Work out the finished part from the listing and answer in its coordinate system (mm). A direction names the side the tool comes from. Round coordinates to 2 decimals unless told otherwise and drop trailing zeros. Order: outer loops, then holes, each group sorted by start corner. A loop starts at its lowest first (then second) coordinate and runs counter-clockwise, first axis right, second up. Notation, with made-up numbers: (-27, 84.25) - (1, 84.25) arc R20 ccw to (1, 103.25) - close; hole circle Ø7 at (10, 38). An arc over 180 degrees is marked (long way). Put each result on its own line as item: value.
```python
from build123d import *

# Parameters (mm, degrees)
BOSS_EXTRU_1_DEPTH           = 22.5
R_P_TITION_CIRCULAIRE2_COUNT = 3
TROU_TARAUD_M51_D            = 4.2
TROU_TARAUD_M51_DEPTH        = 14
TROU_TARAUD_M51_TIP          = 1.2618073
TROU_TARAUD_M52_D            = 4.2
TROU_TARAUD_M52_DEPTH        = 14
TROU_TARAUD_M52_TIP          = 1.2618073
ESQUISSE6_R                  = 4
ESQUISSE6_R_2                = 2.807618462
BOSS_EXTRU_2_DEPTH           = 15


with BuildPart() as part:
    # Esquisse1 → Boss.-Extru.1 (new body, symmetric)
    with BuildSketch(Plane.XY):
        with BuildLine():
            Line((0, 0), (-3.464101615, 2))
            ThreePointArc((-3.464101615, 2), (-2.618614683, 3.023715784), (-1.484614978, 3.714285714))
            ThreePointArc((-1.484614978, 3.714285714), (-1.135374688, 3.722455591), (-0.866025404, 3.5))
            ThreePointArc((-0.866025404, 3.5), (0, 3), (0.866025404, 3.5))
            ThreePointArc((0.866025404, 3.5), (1.135374688, 3.722455591), (1.484614978, 3.714285714))
            ThreePointArc((1.484614978, 3.714285714), (2.618614683, 3.023715784), (3.464101615, 2))
            Line((3.464101615, 2), (0, 0))
        make_face()
    boss_extru_1 = extrude(amount=BOSS_EXTRU_1_DEPTH, both=True)

    # R_p_tition circulaire2: Boss.-Extru.1 ×3 about axis
    r_p_tition_circulaire2_axis = Axis((0, 0, 0), (0, 0, 1))
    for i in range(1, R_P_TITION_CIRCULAIRE2_COUNT):
        add(boss_extru_1.rotate(r_p_tition_circulaire2_axis, i * 360 / R_P_TITION_CIRCULAIRE2_COUNT))

    # Trou taraud_ M51
    with Locations(Plane(origin=(0, 0, -22.5), x_dir=(-1, 0, 0), z_dir=(0, 0, -1))):
        with Locations((0, 0)):
            Hole(TROU_TARAUD_M51_D / 2, depth=TROU_TARAUD_M51_DEPTH)
            with Locations((0, 0, -(TROU_TARAUD_M51_DEPTH + TROU_TARAUD_M51_TIP / 2))):  # 118° drill point
                Cone(0, TROU_TARAUD_M51_D / 2, TROU_TARAUD_M51_TIP, mode=Mode.SUBTRACT)

    # Trou taraud_ M52
    with Locations(Plane.XY.offset(22.5)):
        with Locations((0, 0)):
            Hole(TROU_TARAUD_M52_D / 2, depth=TROU_TARAUD_M52_DEPTH)
            with Locations((0, 0, -(TROU_TARAUD_M52_DEPTH + TROU_TARAUD_M52_TIP / 2))):  # 118° drill point
                Cone(0, TROU_TARAUD_M52_D / 2, TROU_TARAUD_M52_TIP, mode=Mode.SUBTRACT)

    # Esquisse6 → Boss.-Extru.2 (add, symmetric)
    with BuildSketch(Plane.XY):
        with Locations(Location((0, 0, 0), (0, 0, 351.786789298))):  # turned: the seam where the file's is
            Circle(ESQUISSE6_R)
        Circle(ESQUISSE6_R_2, mode=Mode.SUBTRACT)
    extrude(amount=BOSS_EXTRU_2_DEPTH, both=True)


solid = part.part
```
1) Straight lines are drawn through the part: L1, parallel to X at y = 0, z = 13.25; L2, parallel to Z at x = 3, y = -2.5. For each, find the intervals that lie inside material, in ascending order. Write a range as from..to.
Findings below:
L1: x = -4..-2.1, 2.1..4
L2: z = -15..15
2) A cutting plane is placed at B-B on z = -4.5. Write down the section's boundary in (x, y), then the cut area to 3 significant figures.
Findings below:
outline: circle Ø8 at (0, 0)
area: 50.3 mm2
3) Given pin 1 Ø4 at (x, y) = (0, 0) entering from +Z; pin 2 Ø1 at (x, z) = (-1.5, 15) entering from +Y; pin 3 Ø3 at (x, z) = (2.5, -5.5) entering from -Y, each flat-ended and moving along its own axis, determine where each tip first touches the part or whether it passes through.
Findings below:
pin 1: stops at z = 8.44
pin 2: stops at y = 3.87
pin 3: stops at y = -3.87
4) A cutting plane is placed at A-A on z = 13.5. Write down the section's boundary in (x, y).
Findings below:
outline: circle Ø8 at (0, 0); hole circle Ø4.2 at (0, 0)
5) For a pull along X with two mould halves and no side action, classify faces 6 (the cylindrical face through (0, 3, 19)), 7 (the cylindrical face through (-2.6, -1.5, 18.8)), 8 (the cylindrical face through (0, 3, -19)), 9 (the flat face through (3, -2, -15)) as pulls with the +X half, pulls with the -X half, needs draft (parallel to the pull), parting line crosses it, or undercut.
Findings below:
face 6: undercut
face 7: pulls with the -X half
face 8: undercut
face 9: needs draft
6) For faces 1 (the flat face through (0, 3.5, -15)), 2 (the cylindrical face through (-2.003, 0.631, 15.402)), 3 (the cylindrical face through (-2.6, -1.5, -18.7)), 4 (the flat face through (0, 3.5, 15)), 5 (the cylindrical face through (2.6, -1.5, 18.8)), determine the directions among +Z, -Z, +X, -X, +Y, -Y from which every point of the face is accessible in a straight line to the end or side of a thin tool.
Findings below:
face 1: -Z, +Y
face 2: +Z
face 3: -Z, -X
face 4: +Z, +Y
face 5: +Z, +X
